```python
from build123d import *

# Parameters (mm, degrees)
F0_W          = 60
F0_H          = 60
F0_R          = 25
F1_DEPTH      = 30
F2_R          = 12.5
F3_DEPTH      = 25
F3_DEPTH_BACK = 25


with BuildPart() as f1:
    # F0 (on Right) → F1 (new body, symmetric)
    with BuildSketch(Plane.YZ):
        Rectangle(F0_W, F0_H)
        Circle(F0_R, mode=Mode.SUBTRACT)
    extrude(amount=F1_DEPTH, both=True)

    # F2 (on face) → F3 (cut, two sides)
    with BuildSketch(Plane(origin=(0, 0, -30), x_dir=(1, 0, 0), z_dir=(0, 0, -1))) as f3_sk:
        Circle(F2_R)
    extrude(amount=-F3_DEPTH, mode=Mode.SUBTRACT)
    extrude(f3_sk.sketch, amount=-F3_DEPTH_BACK, mode=Mode.SUBTRACT)


solid = f1.part
```
Build history of the part. All positions in model axes, mm. A direction names the side the tool comes from. Round coordinates to 2 decimals unless told otherwise and drop trailing zeros. Order: outer loops, then holes, each group sorted by start corner. A loop starts at its lowest first (then second) coordinate and runs counter-clockwise, first axis right, second up. Notation, with made-up numbers: (61, 59) - (118, 59) arc R17 cw to (118, 66) - close; hole circle Ø3 at (74.5, 37.5). An arc over 180 degrees is marked (long way). Use a Markdown table: item, result.
1) Saw through at B-B on y = 0. Write the cut outline in (x, z), and give its area (3 significant figures).
Recorded:
| item | result |
|---|---|
| outline | (-30, -30) - (-12.5, -30) - (-12.5, -25) - (-30, -25) - close; (-30, 25) - (30, 25) - (30, 30) - (-30, 30) - close; (12.5, -30) - (30, -30) - (30, -25) - (12.5, -25) - close |
| area | 475 mm² |
2) Saw through at C-C on x = 0. Write the cut outline in (y, z), and give its area (3 significant figures).
Recorded:
| item | result |
|---|---|
| outline | (-30, -30) - (-12.5, -30) - (-12.5, -21.65) arc R25 cw (long way) to (12.5, -21.65) - (12.5, -30) - (30, -30) - (30, 30) - (-30, 30) - close |
| area | 1,480 mm² |
3) Wall check: L1, parallel to Y at x = 0, z = -23; L2, parallel to Z at x = -2, y = 0; L3, parallel to Y at x = 4, z = 9. Give the ranges that are in metal, low to high.
Recorded:
| item | result |
|---|---|
| L1 | y = -30 to -12.5, 12.5 to 30 |
| L2 | z = 25 to 30 |
| L3 | y = -30 to -23.32, 23.32 to 30 |
4) Saw through at A-A on z = 0. Write the cut outline in (x, y), and give its area (3 significant figures).
Recorded:
| item | result |
|---|---|
| outline | (-30, -30) - (30, -30) - (30, -25) - (-30, -25) - close; (-30, 25) - (30, 25) - (30, 30) - (-30, 30) - close |
| area | 600 mm² |
5) Saw through at D-D on y = -14. Write the cut outline in (x, z).
Recorded:
| item | result |
|---|---|
| outline | (-30, -30) - (30, -30) - (30, -20.71) - (-30, -20.71) - close; (-30, 20.71) - (30, 20.71) - (30, 30) - (-30, 30) - close |
6) Tool access for faces 1 (the face through (11.923, -3.755, -26.811)), 2 (the face through (0, 30, 0)): list every direction of +Z, -Z, +X, -X, +Y, -Y with a clear straight run to the whole face (end or side of a thin tool).
Recorded:
| item | result |
|---|---|
| face 1 | -Z |
| face 2 | +Z, -Z, +X, -X, +Y |
7) Pull direction Z, two halves, no side cores. Call faces 3 (the face through (30, -27, 0)), 4 (the face through (0, 0, 30)), 5 (the face through (-0.42, -3.255, 24.787)): pulls with the +Z half, pulls with the -Z half, needs draft (parallel to the pull), parting line crosses it, or undercut.
Recorded:
| item | result |
|---|---|
| face 3 | needs draft |
| face 4 | pulls with the +Z half |
| face 5 | undercut |
